CAD build for the part. Positions are in the model's coordinates, mm. Face numbers are marked on the shaded views. A direction names the side the tool comes from. Coordinates: 2 decimals unless noted, no trailing zeros. Write each loop counter-clockwise with the first axis right and the second up, starting at its lowest first coordinate (ties: lowest second). Pieces come first, ordered by that corner, then holes. Notation, with made-up numbers: (38.25, 36.25) - (83.25, 36.25) arc R22 cw to (83.25, 62.25) - close; hole circle Ø3 at (77.5, 79.25). An arc over 180 degrees is marked (long way). One line per question, with ' | ' between items. Start each with the question number.
1. Band-saw the part on B-B, the plane x = 97. Write the cut outline in (y, z).
2. Band-saw the part on D-D, the plane z = -15. Write the cut outline in (x, y).
3. Which spindle directions (+Z, -Z, +X, -X, +Y, -Y) get a long thin tool onto all of the face, cutting with end or side? Do the marked faces 1, 2 and 3. Say none if no direction does.
4. Band-saw the part on A-A, the plane z = 0. Write the cut outline in (x, y), then the cut area to 3 significant figures.
5. Flat gauge pins, fed straight in: P1, Ø16.5, axis at y = 2.5, z = -53.5, coming from the -X side; P2, Ø5, axis at x = 48, y = -2.5, coming from the -Z side; P3, Ø5.5, axis at y = 3, z = -57.5, coming from the -X side; P4, Ø12, axis at x = 78, y = -17.5, coming from the +Z side. Where does each tip first touch, or does it go through?
6. Probe line 1 (Y direction, x = 8, z = 65); line 2 (Y direction, x = 2, z = -55); line 3 (X direction, y = -7.5, z = 22.5). List the from-to ranges inside material, lowest first.
7. Two-plate mould, pull along Z, no slides. Class the marked faces 4, 5 and 6: +Z half, -Z half, draft (parallel to the pull), parting line (faces both ways), or undercut.
8. Band-saw the part on C-C, the plane y = -20. Write the cut outline in (x, z), then the cut area to 3 significant figures.
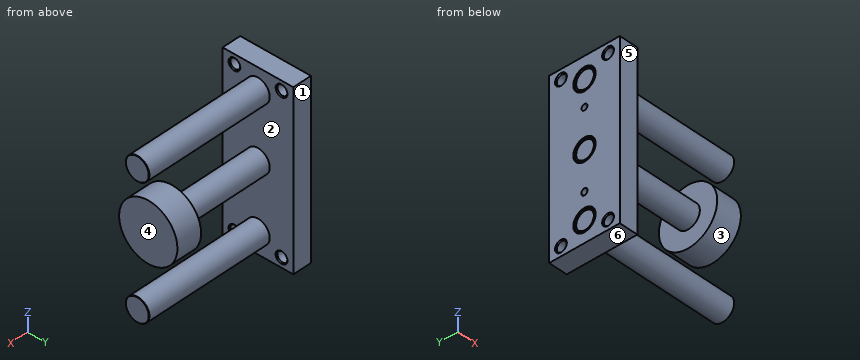
from build123d import *

# Parameters (mm, degrees)
SKETCH_1_W                  = 146
SKETCH_1_H                  = 60
EXTRUDE_1_DEPTH             = 16
PATTERN_LINEAR_1_COUNT      = 3
PATTERN_LINEAR_1_PITCH      = 55
PATTERN_LINEAR_2_COUNT      = 2
PATTERN_LINEAR_2_PITCH      = 130
PATTERN_LINEAR_2_COUNT_DIR2 = 2
PATTERN_LINEAR_2_PITCH_DIR2 = 40
SKETCH_9_W                  = 8
SKETCH_9_H                  = 2.5
HOLE_WIZARD_1_D             = 5
HOLE_WIZARD_1_DEPTH         = 8
HOLE_WIZARD_1_TIP           = 1.443375673
CUT_EXTRUDE_1_DEPTH         = 4


with BuildPart() as part:
    # Sketch 1 → Extrude 1 (new body)
    with BuildSketch(Plane(origin=(0, 0, 0), x_dir=(0, 0, -1), z_dir=(1, 0, 0))):
        Rectangle(SKETCH_1_W, SKETCH_1_H)
    extrude(amount=EXTRUDE_1_DEPTH)

    # Sketch 2 → Cut-Revolve 1 (revolve, cut)
    with BuildSketch(Plane.XY.offset(55), mode=Mode.PRIVATE) as cut_revolve_1_sk:
        Polygon((0, 0), (0, 9.5), (0.5, 9), (6.5, 9), (6.5, 8), (1, 8), (0.5, 7.5), (0.5, 0), align=None)
    cut_revolve_1 = revolve(cut_revolve_1_sk.sketch.rotate(Axis((6.5, 0, 55), (-1, 0, 0)), 270), axis=Axis((6.5, 0, 55), (-1, 0, 0)), mode=Mode.SUBTRACT)

    # Pattern Linear 1: Cut-Revolve 1 ×3
    with Locations(*[(0, 0, -i * PATTERN_LINEAR_1_PITCH) for i in range(1, PATTERN_LINEAR_1_COUNT)]):
        add(cut_revolve_1, mode=Mode.SUBTRACT)

    # Sketch 4 → Revolve 1 (revolve)
    with BuildSketch(Plane.XY, mode=Mode.PRIVATE) as revolve_1_sk:
        Polygon((16, 0), (16, 10), (94.4, 10), (94.4, 24.75), (116, 24.75), (116, 0), align=None)
    revolve(revolve_1_sk.sketch.rotate(Axis((116, 0, 0), (-1, 0, 0)), 270), axis=Axis((116, 0, 0), (-1, 0, 0)))

    # Sketch 5 → Revolve 2 (revolve)
    with BuildSketch(Plane.XY.offset(55), mode=Mode.PRIVATE) as revolve_2_sk:
        Polygon((16, 0), (16, 10), (125.7, 10), (126, 9.7), (126, 0), align=None)
    revolve(revolve_2_sk.sketch.rotate(Axis((126, 0, 55), (-1, 0, 0)), 270), axis=Axis((126, 0, 55), (-1, 0, 0)))

    # Sketch 6 → Revolve 3 (revolve)
    with BuildSketch(Plane.XY.offset(-55), mode=Mode.PRIVATE) as revolve_3_sk:
        Polygon((16, 0), (16, 10), (125.7, 10), (126, 9.7), (126, 0), align=None)
    revolve(revolve_3_sk.sketch.rotate(Axis((126, 0, -55), (-1, 0, 0)), 270), axis=Axis((126, 0, -55), (-1, 0, 0)))

    # Sketch 7 → Cut-Revolve 2 (revolve, cut)
    with BuildSketch(Plane.XY.offset(65), mode=Mode.PRIVATE) as cut_revolve_2_sk:
        Polygon((0, -20), (0, -15), (0.812, -15.812), (15.188, -15.812), (16, -15), (16, -20), align=None)
    cut_revolve_2 = revolve(cut_revolve_2_sk.sketch.rotate(Axis((16, -20, 65), (-1, 0, 0)), 270), axis=Axis((16, -20, 65), (-1, 0, 0)), mode=Mode.SUBTRACT)

    # Pattern Linear 2: Cut-Revolve 2 2 × 2
    with Locations(*[(0, j * PATTERN_LINEAR_2_PITCH_DIR2, -i * PATTERN_LINEAR_2_PITCH) for i in range(PATTERN_LINEAR_2_COUNT) for j in range(PATTERN_LINEAR_2_COUNT_DIR2) if (i, j) != (0, 0)]):
        add(cut_revolve_2, mode=Mode.SUBTRACT)

    # Sketch 9 → Cut-Revolve 3 (revolve, cut)
    with BuildSketch(Plane.XY.offset(33), mode=Mode.PRIVATE) as cut_revolve_3_sk:
        with Locations((4, 1.25)):
            Rectangle(SKETCH_9_W, SKETCH_9_H)
    revolve(cut_revolve_3_sk.sketch.rotate(Axis((8, 0, 33), (-1, 0, 0)), 270), axis=Axis((8, 0, 33), (-1, 0, 0)), mode=Mode.SUBTRACT)

    # Hole Wizard 1
    with Locations(Plane.ZY):
        with Locations((-33, 0)):
            Hole(HOLE_WIZARD_1_D / 2, depth=HOLE_WIZARD_1_DEPTH)
            with Locations((0, 0, -(HOLE_WIZARD_1_DEPTH + HOLE_WIZARD_1_TIP / 2))):  # 120° drill point
                Cone(0, HOLE_WIZARD_1_D / 2, HOLE_WIZARD_1_TIP, mode=Mode.SUBTRACT)

    # Sketch 12 → Cut-Extrude 1 (cut)
    with BuildSketch(Plane(origin=(0, 0, 0), x_dir=(0, 0, -1), z_dir=(1, 0, 0))):
        with BuildLine():
            Line((32.7, -2.5), (33.3, -2.5))
            ThreePointArc((33.3, -2.5), (35.8, 0), (33.3, 2.5))
            Line((33.3, 2.5), (32.7, 2.5))
            ThreePointArc((32.7, 2.5), (30.2, 0), (32.7, -2.5))
        make_face()
    extrude(amount=CUT_EXTRUDE_1_DEPTH, mode=Mode.SUBTRACT)


solid = part.part
Filled in:
1) outline: circle Ø49.5 at (0, 0); circle Ø20 at (0, -55); circle Ø20 at (0, 55)
2) outline: (0, -30) - (16, -30) - (16, 30) - (0, 30) - close; (94.4, -19.69) - (116, -19.69) - (116, 19.69) - (94.4, 19.69) - close
3) face 1: +Z, -Z, +X, -X, +Y | face 2: none | face 3: +X
4) outline: (0, -30) - (16, -30) - (16, -10) - (94.4, -10) - (94.4, -24.75) - (116, -24.75) - (116, 24.75) - (94.4, 24.75) - (94.4, 10) - (16, 10) - (16, 30) - (0, 30) - (0, 9.5) - (0.5, 9) - (6.5, 9) - (6.5, 8) - (1, 8) - (0.5, 7.5) - (0.5, -7.5) - (1, -8) - (6.5, -8) - (6.5, -9) - (0.5, -9) - (0, -9.5) - close | area: 3,580 mm²
5) P1: stops at x = 0 | P2: stops at z = -65 | P3: stops at x = 0.5 | P4: passes through
6) line 1: y = -30 to -24.19, -15.81 to 15.81, 24.19 to 30 | line 2: y = -30 to -9, -8 to 8, 9 to 30 | line 3: x = 0 to 16, 94.4 to 116
7) face 4: undercut | face 5: draft | face 6: -Z half
8) outline: (0, -73) - (16, -73) - (16, -70) - (15.19, -69.19) - (0.81, -69.19) - (0, -70) - close; (0, -60) - (0.81, -60.81) - (15.19, -60.81) - (16, -60) - (16, 60) - (15.19, 60.81) - (0.81, 60.81) - (0, 60) - close; (0, 70) - (0.81, 69.19) - (15.19, 69.19) - (16, 70) - (16, 73) - (0, 73) - close; (94.4, -14.58) - (116, -14.58) - (116, 14.58) - (94.4, 14.58) - close | area: 2,700 mm²
